```python
from build123d import *

# Parameters (mm, degrees)
F0_W     = 723.9
F0_H     = 381
F0_W_2   = 93.000068
F0_H_2   = 93.000068
F0_W_3   = 76.2
F0_H_3   = 76.2
F1_DEPTH = 12.7
F0_R     = 43.18
F2_DEPTH = 10.16
F3_DEPTH = 25.4
F4_DEPTH = 10.16


with BuildPart() as f1:
    # F0 (on Top) → F1 (new body)
    with BuildSketch(Plane.XY):
        with Locations((-11.680007, 37.135195)):
            Rectangle(F0_W, F0_H)
        with Locations((-301.729973, -81.464771)):
            Rectangle(F0_W_2, F0_H_2, mode=Mode.SUBTRACT)
        with Locations((278.369959, -81.464771)):
            Rectangle(F0_W_2, F0_H_2, mode=Mode.SUBTRACT)
        with Locations((159.769993, 37.135195)):
            Rectangle(F0_W_3, F0_H_3, mode=Mode.SUBTRACT)
        with Locations((-301.729973, 37.335093)):
            Rectangle(F0_W_2, F0_H_2, mode=Mode.SUBTRACT)
        with Locations((-301.729973, 155.735161)):
            Rectangle(F0_W_2, F0_H_2, mode=Mode.SUBTRACT)
        with Locations((278.369959, 37.335093)):
            Rectangle(F0_W_2, F0_H_2, mode=Mode.SUBTRACT)
        with Locations((278.369959, 155.735161)):
            Rectangle(F0_W_2, F0_H_2, mode=Mode.SUBTRACT)
    extrude(amount=F1_DEPTH)

    # F0 (on Top) → F2 (join)
    with BuildSketch(Plane.XY):
        with Locations((278.369959, 155.735161)):
            Rectangle(F0_W_2, F0_H_2)
        with Locations((278.369959, 155.735161)):
            Circle(F0_R, mode=Mode.SUBTRACT)
        with Locations((278.369959, 37.335093)):
            Rectangle(F0_W_2, F0_H_2)
        with Locations((278.369959, 37.335093)):
            Circle(F0_R, mode=Mode.SUBTRACT)
        with Locations((278.369959, -81.464771)):
            Rectangle(F0_W_2, F0_H_2)
        with Locations((278.369959, -81.464771)):
            Circle(F0_R, mode=Mode.SUBTRACT)
    extrude(amount=F2_DEPTH)

    # F0 (on Top) → F3 (cut)
    with BuildSketch(Plane.XY):
        with Locations((278.369959, 155.735161)):
            Circle(F0_R)
        with Locations((278.369959, 37.335093)):
            Circle(F0_R)
        with Locations((278.369959, -81.464771)):
            Circle(F0_R)
    extrude(amount=F3_DEPTH, mode=Mode.SUBTRACT)

    # F0 (on Top) → F4 (join)
    with BuildSketch(Plane.XY):
        with Locations((-301.729973, 155.735161)):
            Rectangle(F0_W_2, F0_H_2)
        with Locations((-301.729973, 155.735161)):
            Circle(F0_R, mode=Mode.SUBTRACT)
        with Locations((-301.729973, 37.335093)):
            Rectangle(F0_W_2, F0_H_2)
        with Locations((-301.729973, 37.335093)):
            Circle(F0_R, mode=Mode.SUBTRACT)
        with Locations((-301.729973, -81.464771)):
            Rectangle(F0_W_2, F0_H_2)
        with Locations((-301.729973, -81.464771)):
            Circle(F0_R, mode=Mode.SUBTRACT)
    extrude(amount=F4_DEPTH)


solid = f1.part
```
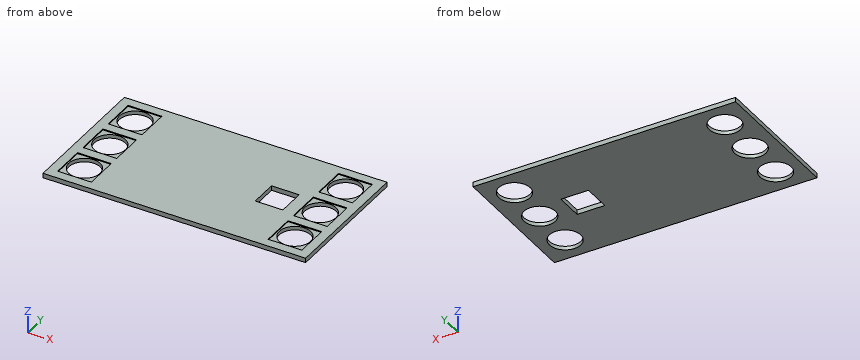
Read the model definition and answer for the solid it produces. Units are mm, in the model's axes. Coordinates: 2 decimals unless noted, no trailing zeros. Write each loop counter-clockwise with the first axis right and the second up, starting at its lowest first coordinate (ties: lowest second). Pieces come first, ordered by that corner, then holes. Notation, with made-up numbers: (88, 89.5) - (107, 89.5) arc R23 cw to (107, 107.5) - close; hole circle Ø10 at (24, 53). An arc over 180 degrees is marked (long way). Answer as a JSON object with one key per item and string values. Group by question number.
1. A cutting plane is placed at D-D (z = 7). Determine the outline of the cut face in (x, y).
2. Consider L1, parallel to X at y = 109.5, z = 10.75; L2, parallel to Y at x = 166.5, z = 7.5; L3, parallel to X at y = 2, z = 5. Determine where each line is inside the solid, lowest interval first. Write a range as [from, to].
3. A cutting plane is placed at C-C (y = 49.5). Determine the outline of the cut face in (x, z).
4. A cutting plane is placed at A-A (y = -101.5). Determine the outline of the cut face in (x, z).
5. A cutting plane is placed at B-B (x = -320). Determine the outline of the cut face in (y, z), plus the area to 3 significant figures.
Worked out:
{
 "1": {"outline": "(-373.63, -153.36) - (350.27, -153.36) - (350.27, 227.64) - (-373.63, 227.64) - close; hole circle Ø86.36 at (-301.73, -81.46); hole circle Ø86.36 at (-301.73, 37.34); hole circle Ø86.36 at (-301.73, 155.74); hole (121.67, -0.96) - (197.87, -0.96) - (197.87, 75.24) - (121.67, 75.24) - close; hole circle Ø86.36 at (278.37, -81.46); hole circle Ø86.36 at (278.37, 37.34); hole circle Ø86.36 at (278.37, 155.74)"},
 "2": {"L1": "x = [-373.63, -348.23], [-255.23, 231.87], [324.87, 350.27]", "L2": "y = [-153.36, -0.96], [75.24, 227.64]", "L3": "x = [-373.63, -326.55], [-276.91, 121.67], [197.87, 253.55], [303.19, 350.27]"},
 "3": {"outline": "(-373.63, 0) - (-343.16, 0) - (-343.16, 10.16) - (-348.23, 10.16) - (-348.23, 12.7) - (-373.63, 12.7) - close; (-260.3, 0) - (121.67, 0) - (121.67, 12.7) - (-255.23, 12.7) - (-255.23, 10.16) - (-260.3, 10.16) - close; (197.87, 0) - (236.94, 0) - (236.94, 10.16) - (231.87, 10.16) - (231.87, 12.7) - (197.87, 12.7) - close; (319.8, 0) - (350.27, 0) - (350.27, 12.7) - (324.87, 12.7) - (324.87, 10.16) - (319.8, 10.16) - close"},
 "4": {"outline": "(-373.63, 0) - (-339.98, 0) - (-339.98, 10.16) - (-348.23, 10.16) - (-348.23, 12.7) - (-373.63, 12.7) - close; (-263.48, 0) - (240.12, 0) - (240.12, 10.16) - (231.87, 10.16) - (231.87, 12.7) - (-255.23, 12.7) - (-255.23, 10.16) - (-263.48, 10.16) - close; (316.62, 0) - (350.27, 0) - (350.27, 12.7) - (324.87, 12.7) - (324.87, 10.16) - (316.62, 10.16) - close"},
 "5": {"outline": "(-153.36, 0) - (-120.59, 0) - (-120.59, 10.16) - (-127.96, 10.16) - (-127.96, 12.7) - (-153.36, 12.7) - close; (-42.34, 0) - (-1.79, 0) - (-1.79, 10.16) - (-9.16, 10.16) - (-9.16, 12.7) - (-34.96, 12.7) - (-34.96, 10.16) - (-42.34, 10.16) - close; (76.46, 0) - (116.61, 0) - (116.61, 10.16) - (109.24, 10.16) - (109.24, 12.7) - (83.84, 12.7) - (83.84, 10.16) - (76.46, 10.16) - close; (194.86, 0) - (227.64, 0) - (227.64, 12.7) - (202.24, 12.7) - (202.24, 10.16) - (194.86, 10.16) - close", "area": "1,750 mm²"}
}
